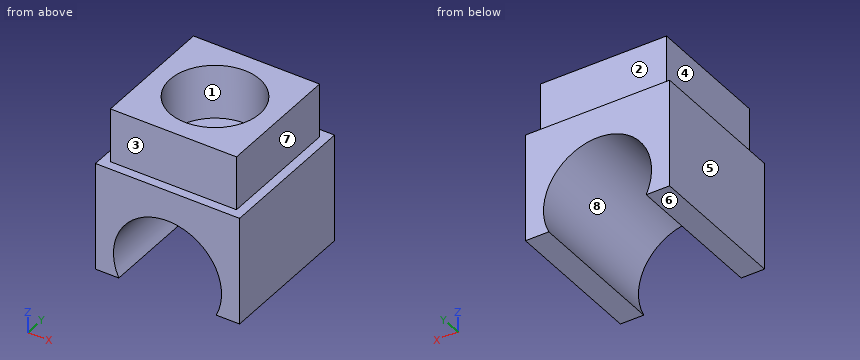
```python
from build123d import *

# Parameters (mm, degrees)
SALIENTE_EXTRUIR1_DEPTH      = 40
SALIENTE_EXTRUIR1_DEPTH_BACK = 40
CROQUIS2_W                   = 70
CROQUIS2_H                   = 70
SALIENTE_EXTRUIR2_DEPTH      = 30
CROQUIS3_R                   = 25
CORTAR_EXTRUIR1_DEPTH        = 30


with BuildPart() as part:
    # Croquis1 → Saliente-Extruir1 (new, two sides: drawn at the far end of the back side and taken through both)
    with BuildSketch(Plane(origin=(0, 0, 0), x_dir=(1, 0, 0), z_dir=(0, 1, 0)).offset(-SALIENTE_EXTRUIR1_DEPTH_BACK)):
        with BuildLine():
            Line((-40, 13), (-27.037011669, 13))
            ThreePointArc((-27.037011669, 13), (0, -30), (27.037011669, 13))
            Line((27.037011669, 13), (40, 13))
            Line((40, 13), (40, -47))
            Line((40, -47), (-40, -47))
            Line((-40, -47), (-40, 13))
        make_face()
    extrude(amount=SALIENTE_EXTRUIR1_DEPTH + SALIENTE_EXTRUIR1_DEPTH_BACK)

    # Croquis2 → Saliente-Extruir2 (add)
    with BuildSketch(Plane.XY.offset(47)):
        Rectangle(CROQUIS2_W, CROQUIS2_H)
    extrude(amount=SALIENTE_EXTRUIR2_DEPTH)

    # Croquis3 → Cortar-Extruir1 (cut)
    with BuildSketch(Plane.XY.offset(77)):
        Circle(CROQUIS3_R)
    extrude(amount=-CORTAR_EXTRUIR1_DEPTH, mode=Mode.SUBTRACT)


solid = part.part
```
CAD build for the part. Positions are in the model's coordinates, mm. Face numbers are marked on the shaded views. A direction names the side the tool comes from. Round coordinates to 2 decimals unless told otherwise and drop trailing zeros. Write each loop counter-clockwise with the first axis right and the second up, starting at its lowest first coordinate (ties: lowest second). Pieces come first, ordered by that corner, then holes. Notation, with made-up numbers: (55, -24.5) - (91, -24.5) arc R30 cw to (91, 4.5) - close; hole circle Ø2 at (-37.75, -5). An arc over 180 degrees is marked (long way). Return JSON: item names as keys, results as strings. Group by question number.
Item 1: 3-axis set-ups, long thin cutter, end or side, ignore diameter. For the marked faces 1, 2, 3 and 4: which of +Z, -Z, +X, -X, +Y, -Y reach the whole face in a straight line?
Item 2: Mould opens along X. For the marked faces 5, 6, 7 and 8 say: +X half, -X half, draft (parallel to the pull), parting line (faces both ways), or undercut.
Item 3: Flat gauge pins, fed straight in: pin 1 Ø15 at (x, z) = (7.5, 59.5) entering from -Y; pin 2 Ø15 at (x, z) = (-13, 62.5) entering from +Y; pin 3 Ø24 at (x, y) = (1, 2) entering from +Z. Where does each tip first touch, or does it go through?
Item 4: Band-saw the part on C-C on x = 0. List the corners of the cut face in (y, z).
Item 5: Probe probe 1 along Y at (x, z) = (0, 57); probe 2 along X at (y, z) = (-24, 0); probe 3 along Z at (x, y) = (0, -23). List the from-to ranges inside material, lowest first.
Item 6: Band-saw the part on D-D on z = 11.5. List the corners of the cut face in (x, y), plus the area to 3 significant figures.
Item 7: Band-saw the part on A-A on z = 0. List the corners of the cut face in (x, y), plus the area to 3 significant figures.
Item 8: Band-saw the part on B-B on y = 0. List the corners of the cut face in (x, z).
Resolved:
{
 "1": {"face 1": "+Z", "face 2": "+Z, +X, -X, +Y", "face 3": "+Z, +X, -X, -Y", "face 4": "+Z, -X, +Y, -Y"},
 "2": {"face 5": "-X half", "face 6": "draft", "face 7": "+X half", "face 8": "undercut"},
 "3": {"pin 1": "stops at y = -35", "pin 2": "stops at y = 35", "pin 3": "stops at z = 47"},
 "4": {"outline": "(-40, 30) - (40, 30) - (40, 47) - (35, 47) - (35, 77) - (25, 77) - (25, 47) - (-25, 47) - (-25, 77) - (-35, 77) - (-35, 47) - (-40, 47) - close"},
 "5": {"probe 1": "y = -35 to -25, 25 to 35", "probe 2": "x = -40 to -30, 30 to 40", "probe 3": "z = 30 to 47"},
 "6": {"outline": "(-40, -40) - (-27.71, -40) - (-27.71, 40) - (-40, 40) - close; (27.71, -40) - (40, -40) - (40, 40) - (27.71, 40) - close", "area": "1,970 mm²"},
 "7": {"outline": "(-40, -40) - (-30, -40) - (-30, 40) - (-40, 40) - close; (30, -40) - (40, -40) - (40, 40) - (30, 40) - close", "area": "1,600 mm²"},
 "8": {"outline": "(-40, -13) - (-27.04, -13) arc R30 cw (long way) to (27.04, -13) - (40, -13) - (40, 47) - (35, 47) - (35, 77) - (25, 77) - (25, 47) - (-25, 47) - (-25, 77) - (-35, 77) - (-35, 47) - (-40, 47) - close"}
}
